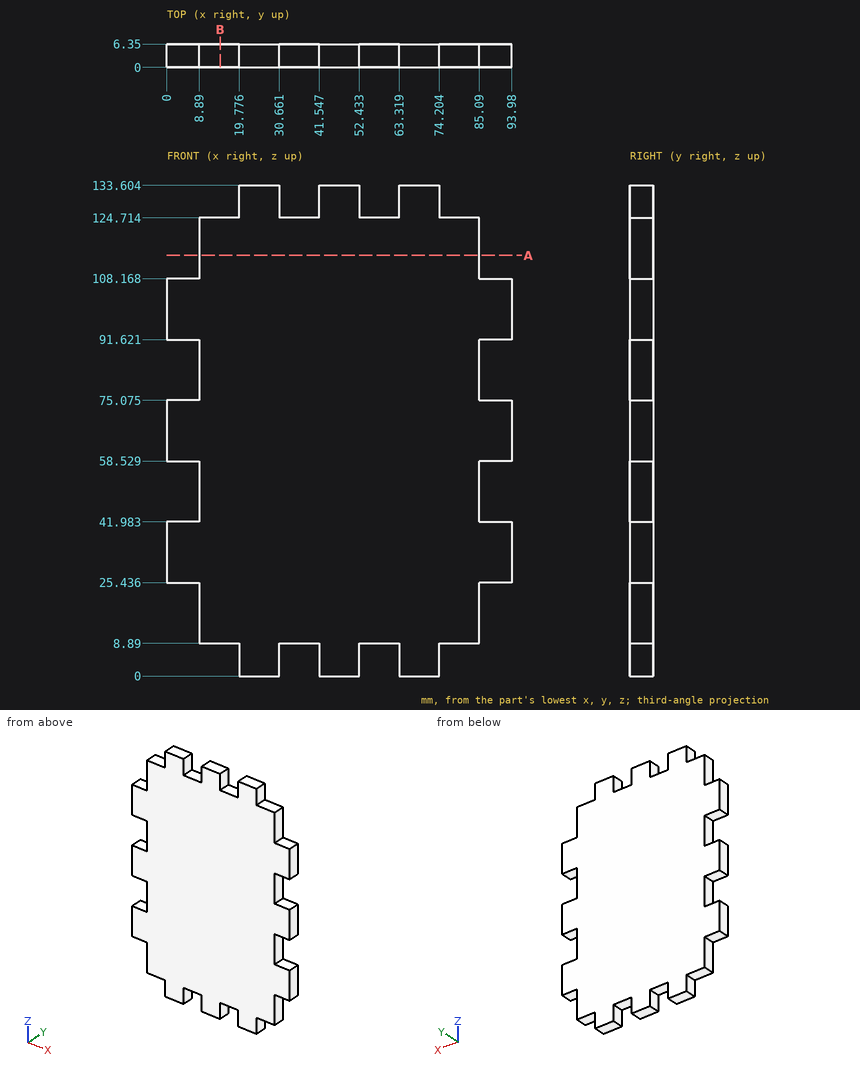
Here's the drawing with two shaded views (mm, measured from the low corner). I have some questions. Coordinates: 2 decimals unless noted, no trailing zeros. Order: outer loops, then holes, each group sorted by start corner. A loop starts at its lowest first (then second) coordinate and runs counter-clockwise, first axis right, second up. Notation, with made-up numbers: (82, 58.5) - (141, 58.5) arc R16 cw to (141, 86.5) - close; hole circle Ø2 at (-14.75, -30). An arc over 180 degrees is marked (long way). Answer in a Markdown table with one row per item. Add a question column.
(1) If we section it at A-A, the plane z = 114.5: Please give me the cut outline in (x, y), then the cut area to 3 significant figures.
(2) If we section it at B-B, the plane x = 14.5: Please give me the cut outline in (y, z).
(3) Will these pins go through, and if not, where does the flat tip stop? pin 1 (3 mm diameter, centred on y = 4, z = 3.5, fed in from +X); pin 2 (1.9 mm diameter, centred on x = 91.5, y = 3, fed in from +Z); pin 3 (3 mm diameter, centred on x = 90, y = 4, fed in from -Z).
(4) I need wall thicknesses on L1, parallel to X at y = 2.75, z = 7.5 (1 decimal); L2, parallel to Z at x = 8.5, y = 4.75 (1 decimal); L3, parallel to X at y = 5, z = 109. Which ranges of each line are inside material? Lowest first, please.
Results are:
| question | item | result |
|---|---|---|
| 1 | outline | (8.89, 0) - (85.09, 0) - (85.09, 6.35) - (8.89, 6.35) - close |
| 1 | area | 484 mm2 |
| 2 | outline | (0, 8.89) - (6.35, 8.89) - (6.35, 124.71) - (0, 124.71) - close |
| 3 | pin 1 | stops at x = 74.2 |
| 3 | pin 2 | stops at z = 108.17 |
| 3 | pin 3 | stops at z = 25.44 |
| 4 | L1 | x = 19.8 to 30.7, 41.5 to 52.4, 63.3 to 74.2 |
| 4 | L2 | z = 25.4 to 42, 58.5 to 75.1, 91.6 to 108.2 |
| 4 | L3 | x = 8.89 to 85.09 |
